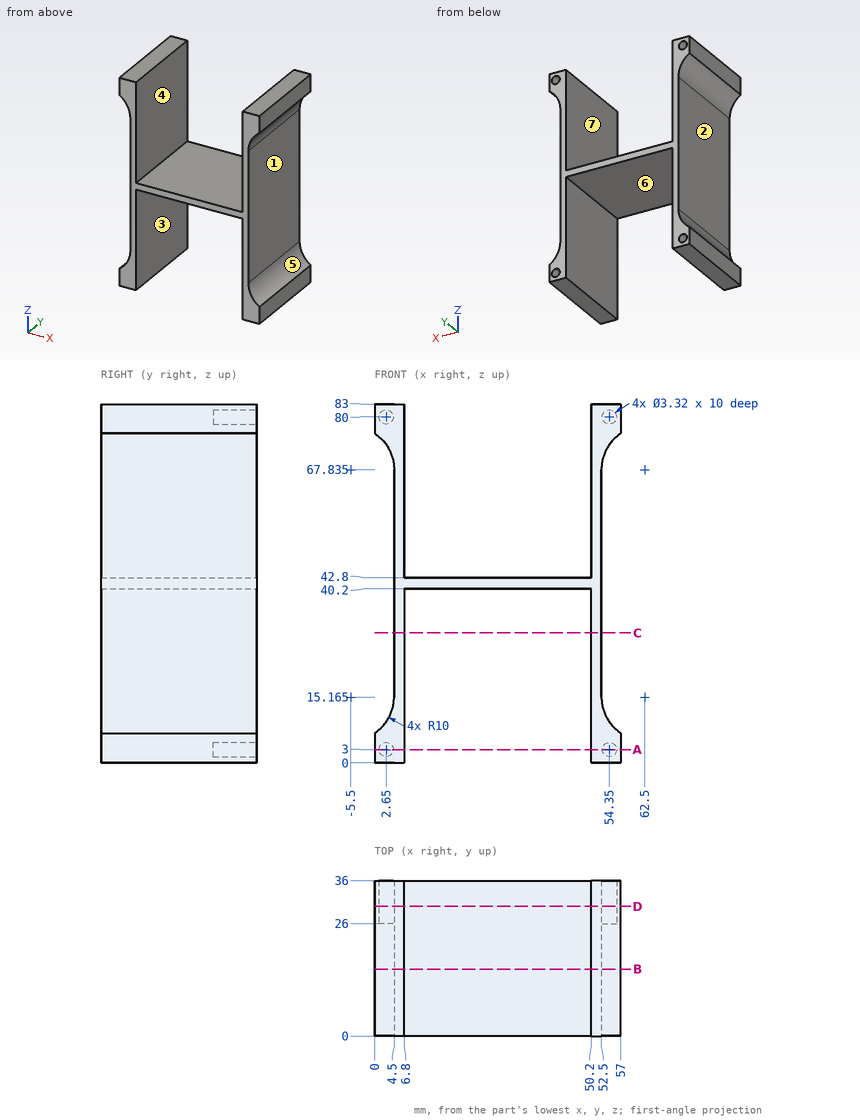
Study the drawing (mm; zero at the part's minimum x, y, z) and answer. A direction names the side the tool comes from. Give positions to 0.01 mm unless a question says otherwise; leave off trailing zeros. Write each loop counter-clockwise with the first axis right and the second up, starting at its lowest first coordinate (ties: lowest second). Pieces come first, ordered by that corner, then holes.
Item 1: Section C-C, the plane z = 30 is taken. Write down the section's boundary in (x, y).
Item 2: Determine the mould class of the marked faces 5, 6 and 7 for opening direction Z: released by +Z, released by -Z, zero draft, split by the parting line, or undercut.
Item 3: Find the intervals of material crossed by line 1 along X through (y, z) = (28.5, 80); line 2 along X through (y, z) = (10.5, 5); line 3 along X through (y, z) = (3, 31), in increasing order.
Item 4: Flat-ended cylindrical pins translate along their axes: P1, Ø10, axis at x = 41.5, y = 30, coming from the -Z side; P2, Ø18, axis at y = 17.5, z = 18, coming from the -X side; P3, Ø2, axis at x = 54.35, z = 3, coming from the +Y side. Find the tip coordinate at first contact, or state that the pin passes through.
Item 5: Section A-A, the plane z = 3 is taken. Write down the section's boundary in (x, y).
Item 6: Which of the six approach directions +Z, -Z, +X, -X, +Y, -Y give full straight-line access (tool end or side, diameter ignored) to the marked faces 1, 2, 3 and 4?
Item 7: Section B-B, the plane y = 15.5 is taken. Write down the section's boundary in (x, z) (1 decimal), plus the area to 3 significant figures.
Item 8: Section D-D, the plane y = 30 is taken. Count the separate pieces of the cut face and the enclosed holes in it, plus the area to 3 significant figures.
Completed:
1. outline: (4.5, 0) - (6.8, 0) - (6.8, 36) - (4.5, 36) - close; (50.2, 0) - (52.5, 0) - (52.5, 36) - (50.2, 36) - close
2. face 5: undercut
2. face 6: released by -Z
2. face 7: zero draft
3. line 1: x = 0 to 0.99, 4.31 to 6.8, 50.2 to 52.69, 56.01 to 57
3. line 2: x = 0 to 6.8, 50.2 to 57
3. line 3: x = 4.5 to 6.8, 50.2 to 52.5
4. P1: stops at z = 40.2
4. P2: stops at x = 2.37
4. P3: stops at y = 26
5. outline: (0, 0) - (6.8, 0) - (6.8, 36) - (4.31, 36) - (4.31, 26) - (0.99, 26) - (0.99, 36) - (0, 36) - close; (50.2, 0) - (57, 0) - (57, 36) - (56.01, 36) - (56.01, 26) - (52.69, 26) - (52.69, 36) - (50.2, 36) - close
6. face 1: +X, +Y, -Y
6. face 2: -X, +Y, -Y
6. face 3: -Z, +Y, -Y
6. face 4: +Z, +Y, -Y
7. outline: (0, 0) - (6.8, 0) - (6.8, 40.2) - (50.2, 40.2) - (50.2, 0) - (57, 0) - (57, 6.8) arc R10 cw to (52.5, 15.2) - (52.5, 67.8) arc R10 cw to (57, 76.2) - (57, 83) - (50.2, 83) - (50.2, 42.8) - (6.8, 42.8) - (6.8, 83) - (0, 83) - (0, 76.2) arc R10 cw to (4.5, 67.8) - (4.5, 15.2) arc R10 cw to (0, 6.8) - close
7. area: 662 mm2
8. separate pieces: 1
8. enclosed holes: 4
8. area: 627 mm2
